The listing builds one solid part. Answer for the finished solid, in the listing's coordinates (mm). Round coordinates to 2 decimals unless told otherwise and drop trailing zeros. Order: outer loops, then holes, each group sorted by start corner. A loop starts at its lowest first (then second) coordinate and runs counter-clockwise, first axis right, second up. Notation, with made-up numbers: (-22, -5.75) - (-18, -5.75) arc R29 cw to (-18, 26.25) - close; hole circle Ø8 at (-35.5, -17). An arc over 180 degrees is marked (long way). Use CSV: the item, a comma, the result in double quotes. Start each with the question number.
Item 1: Flat-ended cylindrical pins translate along their axes: P1, Ø7.5, axis at x = 87, y = 85.5, coming from the +Z side; P2, Ø0.9, axis at x = 10.5, y = -18, coming from the +Z side. Find the tip coordinate at first contact, or state that the pin passes through.
Item 2: Find section B-B, the plane y = -57.5. Give the vertices of the cut face in (x, z).
Item 3: Find section C-C, the plane z = 28. Give the vertices of the cut face in (x, y), plus the area to 3 significant figures.
Item 4: Straight lines are drawn through the part: line 1 along X through (y, z) = (-99, 13); line 2 along X through (y, z) = (-99.5, 3); line 3 along Z through (x, y) = (193, -103.5). For each, find the intervals that lie inside material, in ascending order. Write a range as [from, to].
Item 5: Find section D-D, the plane y = -175. Give the vertices of the cut face in (x, z), plus the area to 3 significant figures.
Item 6: Find section A-A, the plane x = 129. Give the vertices of the cut face in (y, z).
```python
from build123d import *

# Parameters (mm, degrees)
SKETCH2_W           = 309.367
SKETCH2_H           = 311.36
BOSS_EXTRUDE1_DEPTH = 1
SKETCH2_3_R         = 3.5
SKETCH2_3_R_2       = 1.5
SKETCH2_3_R_3       = 4
SKETCH2_3_R_4       = 2
EXTRUDE_THIN1_DEPTH = 20
SKETCH3_R           = 5.5
SKETCH3_R_2         = 1.5
EXTRUDE_THIN2_DEPTH = 35
SKETCH4_W           = 112.631
SKETCH4_H           = 71.36
SKETCH4_W_2         = 163.736
SKETCH4_H_2         = 102.52
SKETCH4_W_3         = 86.868
SKETCH4_H_3         = 64.182745073
SKETCH4_H_4         = 59.613333333
SKETCH4_H_5         = 59.613333334
SKETCH4_W_4         = 183.736
SKETCH4_W_5         = 12.079044756
SKETCH4_H_6         = 69.461977069
SKETCH4_W_6         = 27.221531775
SKETCH4_H_7         = 61.475693889
SKETCH4_W_7         = 27.828675931
SKETCH4_H_8         = 63.062552752
SKETCH4_W_8         = 12
SKETCH4_H_9         = 18.502345826
SKETCH4_W_9         = 12.578204099
SKETCH4_H_10        = 15.179819782
CUT_EXTRUDE1_DEPTH  = 354.494357365


with BuildPart() as part:
    # Sketch2 → Boss-Extrude1 (new body)
    with BuildSketch(Plane.XY):
        with Locations((134.6835, -44.32)):
            Rectangle(SKETCH2_W, SKETCH2_H)
    extrude(amount=BOSS_EXTRUDE1_DEPTH)

    # Sketch2<3> → Extrude-Thin1 (add)
    # profile 1 of 8: a face of its own
    with BuildSketch(Plane.XY):
        with Locations((0, 86.36)):
            Circle(SKETCH2_3_R)
        with Locations((0, 86.36)):
            Circle(SKETCH2_3_R_2, mode=Mode.SUBTRACT)
    # profile 2 of 8: a face of its own
    with BuildSketch(Plane.XY):
        with Locations((86.741, 86.36)):
            Circle(SKETCH2_3_R)
        with Locations((86.741, 86.36)):
            Circle(SKETCH2_3_R_2, mode=Mode.SUBTRACT)
    # profile 3 of 8: a face of its own
    with BuildSketch(Plane.XY):
        Circle(SKETCH2_3_R)
        Circle(SKETCH2_3_R_2, mode=Mode.SUBTRACT)
    # profile 4 of 8: a face of its own
    with BuildSketch(Plane.XY):
        with Locations((86.741, 0)):
            Circle(SKETCH2_3_R)
        with Locations((86.741, 0)):
            Circle(SKETCH2_3_R_2, mode=Mode.SUBTRACT)
    # profile 5 of 8: a face of its own
    with BuildSketch(Plane.XY):
        with Locations((95.631, -1.16)):
            Circle(SKETCH2_3_R_3)
        with Locations((95.631, -1.16)):
            Circle(SKETCH2_3_R_4, mode=Mode.SUBTRACT)
    # profile 6 of 8: a face of its own
    with BuildSketch(Plane.XY):
        with Locations((95.631, 86.61)):
            Circle(SKETCH2_3_R_3)
        with Locations((95.631, 86.61)):
            Circle(SKETCH2_3_R_4, mode=Mode.SUBTRACT)
    # profile 7 of 8: a face of its own
    with BuildSketch(Plane.XY):
        with Locations((269.367, 86.61)):
            Circle(SKETCH2_3_R_3)
        with Locations((269.367, 86.61)):
            Circle(SKETCH2_3_R_4, mode=Mode.SUBTRACT)
    # profile 8 of 8: a face of its own
    with BuildSketch(Plane.XY):
        with Locations((269.367, -1.16)):
            Circle(SKETCH2_3_R_3)
        with Locations((269.367, -1.16)):
            Circle(SKETCH2_3_R_4, mode=Mode.SUBTRACT)
    extrude(amount=EXTRUDE_THIN1_DEPTH)

    # Sketch3 → Extrude-Thin2 (add)
    # profile 1 of 4: a face of its own
    with BuildSketch(Plane.XY.offset(1)):
        with Locations((10, -18)):
            Circle(SKETCH3_R)
        with Locations((10, -18)):
            Circle(SKETCH3_R_2, mode=Mode.SUBTRACT)
    # profile 2 of 4: a face of its own
    with BuildSketch(Plane.XY.offset(1)):
        with Locations((10, -99)):
            Circle(SKETCH3_R)
        with Locations((10, -99)):
            Circle(SKETCH3_R_2, mode=Mode.SUBTRACT)
    # profile 3 of 4: a face of its own
    with BuildSketch(Plane.XY.offset(1)):
        with Locations((10, -109)):
            Circle(SKETCH3_R)
        with Locations((10, -109)):
            Circle(SKETCH3_R_2, mode=Mode.SUBTRACT)
    # profile 4 of 4: a face of its own
    with BuildSketch(Plane.XY.offset(1)):
        with Locations((10, -190)):
            Circle(SKETCH3_R)
        with Locations((10, -190)):
            Circle(SKETCH3_R_2, mode=Mode.SUBTRACT)
    extrude(amount=EXTRUDE_THIN2_DEPTH)

    # Sketch4 → Cut-Extrude1 (cut, through all)
    with BuildSketch(Plane.XY.offset(1)):
        with Locations((39.3155, 45.68)):
            Rectangle(SKETCH4_W, SKETCH4_H)
        with Locations((182.499, 55.1)):
            Rectangle(SKETCH4_W_2, SKETCH4_H_2)
        with Locations((144.065, -33.681960797)):
            Rectangle(SKETCH4_W_3, SKETCH4_H_3)
        with Locations((240.933, -35.966666667)):
            Rectangle(SKETCH4_W_3, SKETCH4_H_4)
        with Locations((144.065, -100.58)):
            Rectangle(SKETCH4_W_3, SKETCH4_H_5)
        with Locations((240.933, -100.58)):
            Rectangle(SKETCH4_W_3, SKETCH4_H_5)
        with BuildLine():
            Line((20, 5), (74.440730541, 5))
            ThreePointArc((74.440730541, 5), (79.116741885, -10.87047915), (95.631, -9.862278071))
            Line((95.631, -9.862278071), (95.631, -195))
            Line((95.631, -195), (20, -195))
            Line((20, -195), (20, 5))
        make_face()
        with Locations((192.499, -165.193333333)):
            Rectangle(SKETCH4_W_4, SKETCH4_H_4)
        Polygon((8.304053723, 103.951159657), (78.368777901, 103.951159657), (78.368777901, 87.023616947), (8.304053723, 87.023616947), (8.304053723, 95.487388302), (-13.644840997, 95.487388302), (-13.644840997, 103.951159657), align=None)
        with Locations((278.577905398, 42.236447079)):
            Rectangle(SKETCH4_W_5, SKETCH4_H_6)
        with Locations((1.610765888, -151.832307187)):
            Rectangle(SKETCH4_W_6, SKETCH4_H_7)
        with Locations((1.914337966, -57.002403063)):
            Rectangle(SKETCH4_W_7, SKETCH4_H_8)
        with Locations((-6, -104.251172913)):
            Rectangle(SKETCH4_W_8, SKETCH4_H_9)
        with Locations((-6.28910205, -13.749909891)):
            Rectangle(SKETCH4_W_9, SKETCH4_H_10)
    extrude(amount=-CUT_EXTRUDE1_DEPTH, mode=Mode.SUBTRACT)


solid = part.part
```
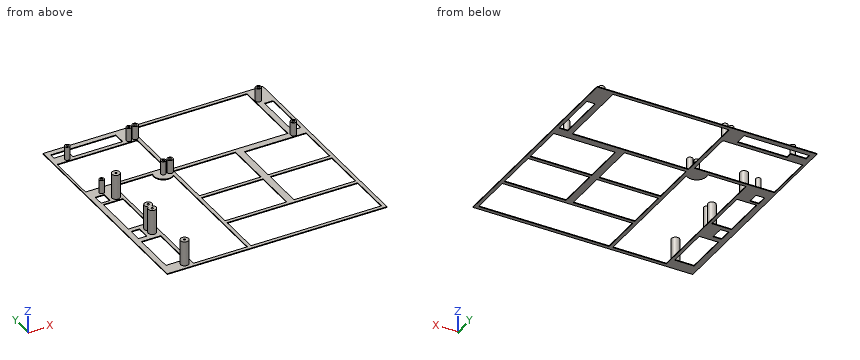
Worked out:
1,P1,"stops at z = 20"
1,P2,"stops at z = 1"
2,outline,"(-20, 0) - (-12, 0) - (-12, 1) - (-20, 1) - close; (15.83, 0) - (20, 0) - (20, 1) - (15.83, 1) - close; (95.63, 0) - (100.63, 0) - (100.63, 1) - (95.63, 1) - close; (187.5, 0) - (197.5, 0) - (197.5, 1) - (187.5, 1) - close; (284.37, 0) - (289.37, 0) - (289.37, 1) - (284.37, 1) - close"
3,outline,"circle Ø11 at (10, -190); circle Ø11 at (10, -18); (7.71, -104) arc R5.5 ccw (long way) to (12.29, -104) arc R5.5 ccw (long way) to start; hole circle Ø3 at (10, -190); hole circle Ø3 at (10, -109); hole circle Ø3 at (10, -99); hole circle Ø3 at (10, -18)"
3,area,"349 mm²"
4,line 1,"x = [4.5, 8.5], [11.5, 15.5]"
4,line 2,"x = [4.52, 8.59], [11.41, 15.48]"
4,line 3,"z = [0, 1]"
5,outline,"(-20, 0) - (-12, 0) - (-12, 1) - (-20, 1) - close; (15.22, 0) - (20, 0) - (20, 1) - (15.22, 1) - close; (95.63, 0) - (100.63, 0) - (100.63, 1) - (95.63, 1) - close; (284.37, 0) - (289.37, 0) - (289.37, 1) - (284.37, 1) - close"
5,area,"22.8 mm²"
6,outline,"(-200, 0) - (-195, 0) - (-195, 1) - (-200, 1) - close; (-135.39, 0) - (-130.39, 0) - (-130.39, 1) - (-135.39, 1) - close; (-70.77, 0) - (-65.77, 0) - (-65.77, 1) - (-70.77, 1) - close; (-1.59, 0) - (3.84, 0) - (3.84, 1) - (-1.59, 1) - close; (106.36, 0) - (111.36, 0) - (111.36, 1) - (106.36, 1) - close"
